from build123d import *

# Parameters (mm, degrees)
BOSS_EXTRUDE1_DEPTH = 20
SKETCH2_R           = 2.75
SKETCH2_R_2         = 3.05
CUT_EXTRUDE1_DEPTH  = 40.553760883
BOSS_EXTRUDE2_START = 4
SKETCH3_W           = 20
SKETCH3_H           = 20
SKETCH3_R           = 3.05
BOSS_EXTRUDE2_DEPTH = 4
FILLET1_R           = 2


with BuildPart() as part:
    # Sketch1 → Boss-Extrude1 (new body)
    with BuildSketch(Plane.XY):
        Polygon((-10.25, 1.5), (10.25, 1.5), (10.25, 21.5), (13.25, 21.5), (13.25, -21), (10.25, -21), (10.25, -1.5), (-10.25, -1.5), (-10.25, -21), (-13.25, -21), (-13.25, 21.5), (-10.25, 21.5), align=None)
    extrude(amount=BOSS_EXTRUDE1_DEPTH)

    # Sketch2 → Cut-Extrude1 (cut, through all)
    with BuildSketch(Plane(origin=(13.25, 0, 0), x_dir=(0, 0, -1), z_dir=(1, 0, 0))):
        with Locations(Location((-10, -11.5, 0), (0, 0, 90))):
            Circle(SKETCH2_R)
        with Locations(Location((-10, 16.5, 0), (0, 0, 90))):
            Circle(SKETCH2_R_2)
    extrude(amount=-CUT_EXTRUDE1_DEPTH, mode=Mode.SUBTRACT)

    # Sketch3 → Boss-Extrude2 (add)
    with BuildSketch(Plane(origin=(-10.25, 0, 0), x_dir=(0, 0, -1), z_dir=(1, 0, 0)).offset(BOSS_EXTRUDE2_START)):
        with Locations((-10, 11.5)):
            Rectangle(SKETCH3_W, SKETCH3_H)
        with Locations(Location((-10, 16.5, 0), (0, 0, 90))):
            Circle(SKETCH3_R, mode=Mode.SUBTRACT)
    extrude(amount=-BOSS_EXTRUDE2_DEPTH)

    # Fillet1
    fillet1_edges = [part.edges().sort_by_distance(p)[0] for p in [
        (-9.75, 21.5, 0),
        (11.75, 21.5, 0),
        (11.75, -21, 0),
        (-11.75, -21, 0),
        (11.75, -21, 20),
        (11.75, 21.5, 20),
        (-9.75, 21.5, 20),
        (-11.75, -21, 20),
    ]]
    fillet(fillet1_edges, radius=FILLET1_R)


solid = part.part
Source: CAD feature listing. Evaluate the final solid. Frame: model axes, mm. A direction names the side the tool comes from. Round coordinates to 2 decimals unless told otherwise and drop trailing zeros. Write each loop counter-clockwise with the first axis right and the second up, starting at its lowest first coordinate (ties: lowest second). Pieces come first, ordered by that corner, then holes. Notation, with made-up numbers: M 68.5,84.25 L 110.5,84.25 A17 cw 110.5,92.25 Z; hole C -18.5,-20 d11. An arc over 180 degrees is marked long. One line per item, written item: value. Start each with the question number.
Item 1: Mould query, pull axis Y, two halves, no side actions, for faces 4 (the cylindrical face through (-11.77, -20.4, 0.57)), 5 (the cylindrical face through (-9.7, 18.14, 12.57)), 6 (the flat face through (-6.25, 12, 10)), 7 (the cylindrical face through (-11.73, -10.02, 12.32)). Classes: pulls with the +Y half, pulls with the -Y half, needs draft (parallel to the pull), parting line crosses it, or undercut.
Item 2: Section query A-A (y = -5). Return the cut outline in (x, z), plus the area to 3 significant figures.
Item 3: Set-up query: faces 1 (the flat face through (10.25, 11, 10)), 2 (the flat face through (0, -1.5, 10)), 3 (the cylindrical face through (11.77, -10.02, 12.32)). Return all of +Z, -Z, +X, -X, +Y, -Y with unobstructed straight access to the full face (end or side cutting, diameter ignored); none if empty.
Item 4: Section query D-D (x = -11.5). Return the cut outline in (y, z), plus the area to 3 significant figures.
Item 5: Ray query, L1, parallel to X at y = 6.5, z = 2.75; L2, parallel to X at y = -16, z = 17.5; L3, parallel to Z at x = -11.15, y = -11.5. Return the intervals inside material, ascending. Write a range as from..to.
Item 6: Section query C-C (y = 16.5). Return the cut outline in (x, z), plus the area to 3 significant figures.
Item 7: Section query B-B (z = 10). Return the cut outline in (x, y).
Item 8: Pin query (flat end, axial travel): pin 1 (1.5 mm diameter, centred on x = -5.5, z = 8.5, fed in from -Y); pin 2 (4 mm diameter, centred on x = 8, z = 9.5, fed in from +Y). Return the tip coordinate at first contact, or that it passes through.
Result set:
1. face 4: pulls with the -Y half
1. face 5: undercut
1. face 6: needs draft
1. face 7: undercut
2. outline: M -13.25,0 L -10.25,0 L -10.25,20 L -13.25,20 Z; M 10.25,0 L 13.25,0 L 13.25,20 L 10.25,20 Z
2. area: 120 mm²
3. face 1: +Z, -Z, +Y
3. face 2: +Z, -Z, -Y
3. face 3: +X, -X
4. outline: M -21,2 A2 ccw -19,0 L 19.5,0 A2 ccw 21.5,2 L 21.5,18 A2 ccw 19.5,20 L -19,20 A2 ccw -21,18 Z; hole C -11.5,10 d5.5; hole C 16.5,10 d6.1
4. area: 794 mm²
5. L1: x = -13.25..-6.25, 10.25..13.25
5. L2: x = -13.25..-10.25, 10.25..13.25
5. L3: z = 0..7.25, 12.75..20
6. outline: M -13.25,0 L -6.25,0 L -6.25,6.95 L -13.25,6.95 Z; M -13.25,13.05 L -6.25,13.05 L -6.25,20 L -13.25,20 Z; M 10.25,0 L 13.25,0 L 13.25,6.95 L 10.25,6.95 Z; M 10.25,13.05 L 13.25,13.05 L 13.25,20 L 10.25,20 Z
6. area: 139 mm²
7. outline: M -13.25,-21 L -10.25,-21 L -10.25,-14.25 L -13.25,-14.25 Z; M -13.25,-8.75 L -10.25,-8.75 L -10.25,-1.5 L 10.25,-1.5 L 10.25,-8.75 L 13.25,-8.75 L 13.25,13.45 L 10.25,13.45 L 10.25,1.5 L -6.25,1.5 L -6.25,13.45 L -13.25,13.45 Z; M -13.25,19.55 L -6.25,19.55 L -6.25,21.5 L -13.25,21.5 Z; M 10.25,-21 L 13.25,-21 L 13.25,-14.25 L 10.25,-14.25 Z; M 10.25,19.55 L 13.25,19.55 L 13.25,21.5 L 10.25,21.5 Z
8. pin 1: stops at y = -1.5
8. pin 2: stops at y = 1.5
